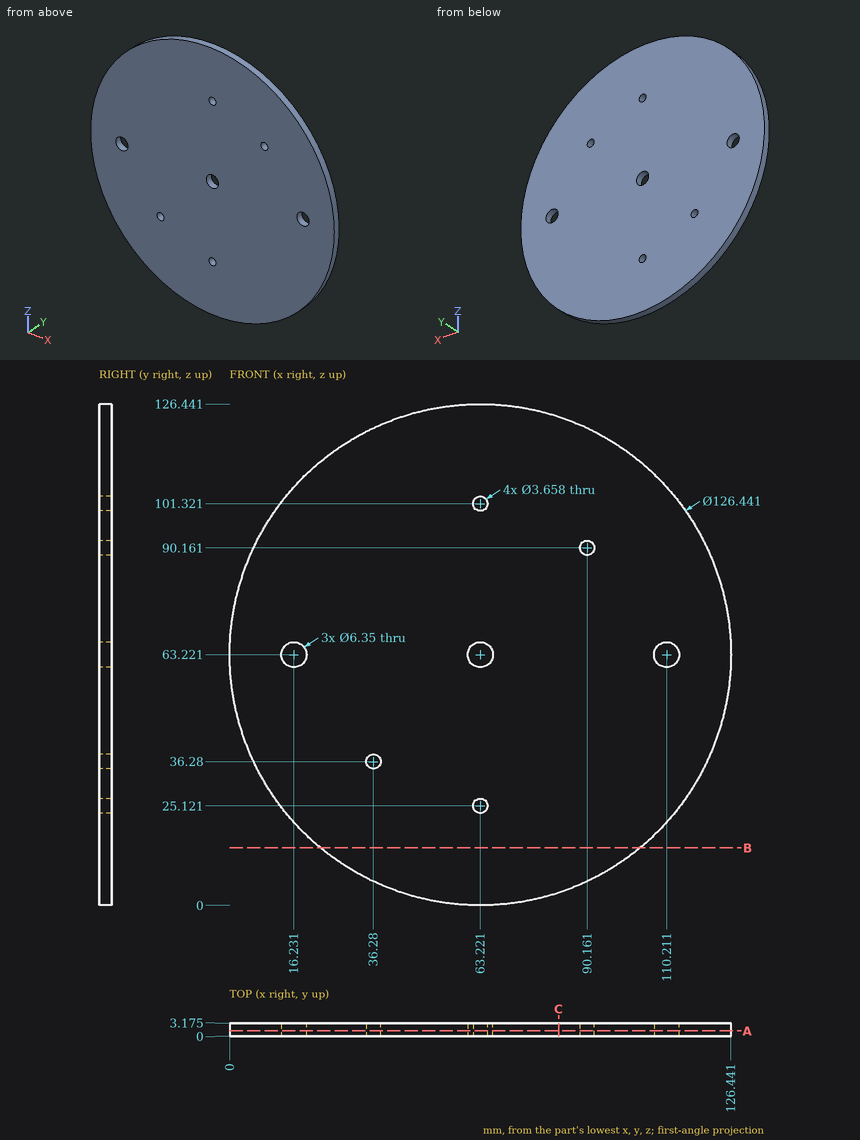
Could you check a few things on this drawing? It's one solid part, dimensions in mm from its lowest x, y, z. Coordinates: 2 decimals unless noted, no trailing zeros. Loops run counter-clockwise (first coordinate to the right, second up) from the corner with the lowest first, then second, coordinate; pieces in that order, holes last.
1. Imagine slicing it at A-A (y = 1.3). Give the number of separate pieces and of enclosed holes in the cut face, and give its area (3 significant figures).
2. Imagine slicing it at B-B (z = 14.5). Please give me the cut outline in (x, y) (1 decimal).
3. Imagine slicing it at C-C (x = 83). Please give me the cut outline in (y, z) (1 decimal).
4. For P1, Ø1, axis at x = 104, z = 94, coming from the -Y side, with a flat end and sliding along its axis, tell me the tip position at first contact or that it passes through.
5. I need wall thicknesses on L1, parallel to X at y = 1.3, z = 64.5 (1 decimal); L2, parallel to X at y = 0.85, z = 61.5 (1 decimal); L3, parallel to Z at x = 64, y = 0.4 (1 decimal). Which ranges of each line are inside material? Lowest first, please.
Computed values:
1. separate pieces: 1
1. enclosed holes: 7
1. area: 12,400 mm2
2. outline: (22.9, 0) - (103.5, 0) - (103.5, 3.2) - (22.9, 3.2) - close
3. outline: (0, 3.2) - (3.2, 3.2) - (3.2, 123.3) - (0, 123.3) - close
4. P1: stops at y = 0
5. L1: x = 0 to 13.3, 19.1 to 60.3, 66.1 to 107.3, 113.1 to 126.4
5. L2: x = 0 to 13.6, 18.9 to 60.6, 65.9 to 107.5, 112.9 to 126.4
5. L3: z = 0 to 23.5, 26.8 to 60.1, 66.3 to 99.7, 103 to 126.4
